Input: part model. Units: mm. Frame: model coordinates. Coordinates: 2 decimals unless noted, no trailing zeros. Order: outer loops, then holes, each group sorted by start corner. A loop starts at its lowest first (then second) coordinate and runs counter-clockwise, first axis right, second up. Notation, with made-up numbers: M -11.75,-40 L -2.75,-40 A25 cw -2.75,-26 Z; hole C -11,-9.5 d8. An arc over 180 degrees is marked long. Answer in a Markdown table with one row per item.
from build123d import *

# Parameters (mm, degrees)
F0_W     = 24
F0_H     = 24
F1_DEPTH = 9.5
F2_R     = 4.5
F4_R     = 8
F5_DEPTH = 9.501
F3_R     = 1.35
F6_DEPTH = 9.501


with BuildPart() as f1:
    # F0 (on Top) → F1 (new body)
    with BuildSketch(Plane.XY):
        with Locations((12, 12)):
            Rectangle(F0_W, F0_H)
    extrude(amount=F1_DEPTH)

    # F2
    f2_edges = [f1.edges().sort_by_distance(p)[0] for p in [
        (0, 0, 4.75),
        (24, 0, 4.75),
        (24, 24, 4.75),
        (0, 24, 4.75),
    ]]
    fillet(f2_edges, radius=F2_R)

    # F4 (on face) → F5 (cut, through all)
    with BuildSketch(Plane.XY.offset(9.5)):
        with Locations((12, 12)):
            Circle(F4_R)
    extrude(amount=-F5_DEPTH, mode=Mode.SUBTRACT)

    # F3 (on face) → F6 (cut, through all)
    with BuildSketch(Plane.XY.offset(9.5)):
        with Locations((4, 4)):
            Circle(F3_R)
        with Locations((4, 20)):
            Circle(F3_R)
        with Locations((20, 4)):
            Circle(F3_R)
        with Locations((20, 20)):
            Circle(F3_R)
    extrude(amount=-F6_DEPTH, mode=Mode.SUBTRACT)


solid = f1.part
1) Cut plane D-D, the plane y = 13. Output: boundary loops of the cut face in (x, z).
Resolved:
| item | result |
|---|---|
| outline | M 0,0 L 4.06,0 L 4.06,9.5 L 0,9.5 Z; M 19.94,0 L 24,0 L 24,9.5 L 19.94,9.5 Z |
2) Cut plane B-B, the plane z = 4.5. Output: boundary loops of the cut face in (x, y), and give its area (3 significant figures).
Resolved:
| item | result |
|---|---|
| outline | M 0,4.5 A4.5 ccw 4.5,0 L 19.5,0 A4.5 ccw 24,4.5 L 24,19.5 A4.5 ccw 19.5,24 L 4.5,24 A4.5 ccw 0,19.5 Z; hole C 4,4 d2.7; hole C 4,20 d2.7; hole C 12,12 d16; hole C 20,4 d2.7; hole C 20,20 d2.7 |
| area | 335 mm2 |
3) Material intervals for probe 1 along Y at (x, z) = (12.25, 2.5); probe 2 along Y at (x, z) = (10.75, 1.5), sorted ascending.
Resolved:
| item | result |
|---|---|
| probe 1 | y = 0 to 4, 20 to 24 |
| probe 2 | y = 0 to 4.1, 19.9 to 24 |
4) Cut plane A-A, the plane x = 12. Output: boundary loops of the cut face in (y, z), and give its area (3 significant figures).
Resolved:
| item | result |
|---|---|
| outline | M 0,0 L 4,0 L 4,9.5 L 0,9.5 Z; M 20,0 L 24,0 L 24,9.5 L 20,9.5 Z |
| area | 76.0 mm2 |
5) Contact query for flat-ended pins moving along their axis: pin 1 (1.6 mm diameter, centred on x = 4, y = 20, fed in from +Z); pin 2 (1 mm diameter, centred on x = 20.5, z = 8.5, fed in from -Y); pin 3 (5 mm diameter, centred on x = 14, y = 18, fed in from -Z). Output: stop coordinate, or through.
Resolved:
| item | result |
|---|---|
| pin 1 | passes through |
| pin 2 | stops at y = 0.03 |
| pin 3 | stops at z = 0 |
6) Cut plane C-C, the plane y = 3. Output: boundary loops of the cut face in (x, z), and give its area (3 significant figures).
Resolved:
| item | result |
|---|---|
| outline | M 0.26,0 L 3.09,0 L 3.09,9.5 L 0.26,9.5 Z; M 4.91,0 L 19.09,0 L 19.09,9.5 L 4.91,9.5 Z; M 20.91,0 L 23.74,0 L 23.74,9.5 L 20.91,9.5 Z |
| area | 189 mm2 |
7) Mould query, pull axis Y, two halves, no side actions, for faces 1 (the face through (21.247, 19.483, 4.816)), 2 (the face through (1.283, 1.353, 4.816)), 3 (the face through (0, 12, 5)). Classes: +Y half, -Y half, draft (parallel to the pull), parting line (faces both ways), or undercut.
Resolved:
| item | result |
|---|---|
| face 1 | undercut |
| face 2 | -Y half |
| face 3 | draft |
